For this review, take the finished solid that the model builds, in its own axes (mm). Face numbers are marked on the shaded views. A direction names the side the tool comes from. Give positions to 0.01 mm unless a question says otherwise; leave off trailing zeros. Loops run counter-clockwise (first coordinate to the right, second up) from the corner with the lowest first, then second, coordinate; pieces in that order, holes last. Notation, with made-up numbers: (17.5, 89) - (74.5, 89) arc R10 cw to (74.5, 96) - close; hole circle Ø3 at (-13, 57). An arc over 180 degrees is marked (long way). Answer as CSV lines item,"result".
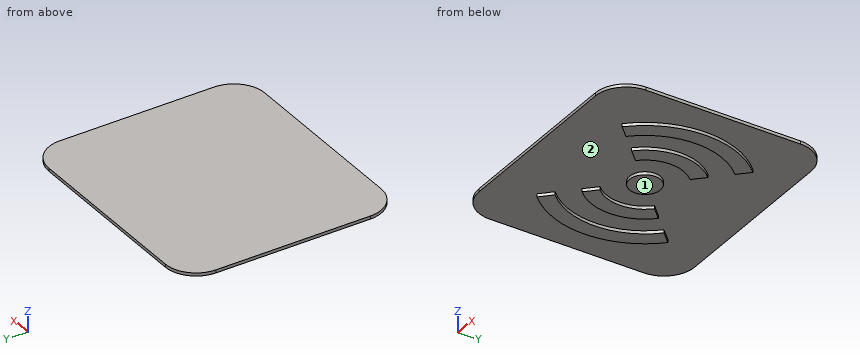
from build123d import *

# Parameters (mm, degrees)
SKETCH1_W           = 78
SKETCH1_H           = 70
BOSS_EXTRUDE1_DEPTH = 1
FILLET1_R           = 10
SKETCH2_R           = 5
BOSS_EXTRUDE3_DEPTH = 1


with BuildPart() as part:
    # Sketch1 → Boss-Extrude1 (new body)
    with BuildSketch(Plane.XY):
        with Locations((-0.075399098, 4.950190099)):
            Rectangle(SKETCH1_W, SKETCH1_H)
    extrude(amount=BOSS_EXTRUDE1_DEPTH)

    # Fillet1
    fillet1_edges = [part.edges().sort_by_distance(p)[0] for p in [
        (38.924600902, -30.049809901, 0.5),
        (-39.075399098, -30.049809901, 0.5),
        (-39.075399098, 39.950190099, 0.5),
        (38.924600902, 39.950190099, 0.5),
    ]]
    fillet(fillet1_edges, radius=FILLET1_R)

    # Sketch2 → Boss-Extrude3 (add)
    with BuildSketch(Plane(origin=(0, 0, 0), x_dir=(-1, 0, 0), z_dir=(0, 0, -1))):
        with BuildLine():
            Line((12.449767768, -7.424178572), (8.914233862, -3.888644666))
            ThreePointArc((8.914233862, -3.888644666), (12.575399098, 4.950190099), (8.914233862, 13.789024864))
            Line((8.914233862, 13.789024864), (12.449767768, 17.32455877))
            ThreePointArc((12.449767768, 17.32455877), (17.575399098, 4.950190099), (12.449767768, -7.424178572))
        make_face()
        with Locations(Location((0.075399098, 4.950190099, 0), (0, 0, 180))):
            Circle(SKETCH2_R)
        with BuildLine():
            Line((21.288602533, -16.263013337), (17.753068627, -12.727479431))
            ThreePointArc((17.753068627, -12.727479431), (25.075399098, 4.950190099), (17.753068627, 22.627859629))
            Line((17.753068627, 22.627859629), (21.288602533, 26.163393535))
            ThreePointArc((21.288602533, 26.163393535), (30.075399098, 4.950190099), (21.288602533, -16.263013337))
        make_face()
        with BuildLine():
            Line((-12.298969573, -7.424178572), (-8.763435667, -3.888644666))
            ThreePointArc((-8.763435667, -3.888644666), (-12.424600902, 4.950190099), (-8.763435667, 13.789024864))
            Line((-8.763435667, 13.789024864), (-12.298969573, 17.32455877))
            ThreePointArc((-12.298969573, 17.32455877), (-17.424600902, 4.950190099), (-12.298969573, -7.424178572))
        make_face()
        with BuildLine():
            Line((-21.137804338, -16.263013337), (-17.602270432, -12.727479431))
            ThreePointArc((-17.602270432, -12.727479431), (-24.924600902, 4.950190099), (-17.602270432, 22.627859629))
            Line((-17.602270432, 22.627859629), (-21.137804338, 26.163393535))
            ThreePointArc((-21.137804338, 26.163393535), (-29.924600902, 4.950190099), (-21.137804338, -16.263013337))
        make_face()
    extrude(amount=BOSS_EXTRUDE3_DEPTH)


solid = part.part
1) Consider section C-C on y = 21. Write out the cut boundary in (x, z).
From the geometry:
outline,"(-39.08, 0) - (-25.42, 0) - (-25.42, -1) - (-19.24, -1) - (-19.24, 0) - (19.09, 0) - (19.09, -1) - (25.27, -1) - (25.27, 0) - (38.92, 0) - (38.92, 1) - (-39.08, 1) - close"
2) Wall thickness on line 1 (X direction, y = 10.5, z = -0.6); line 2 (X direction, y = -12, z = -0.35); line 3 (Z direction, x = 20.5, y = -27): over which ranges is each line inside the solid? List them lowest first. Write a range as from..to.
From the geometry:
line 1,"x = -29.56..-24.45, -16.67..-11.28, 11.13..16.52, 24.3..29.41"
line 2,"x = -24.83..-18.45, 18.3..24.68"
line 3,"z = 0..1"
3) Consider section B-B on x = -4. Write out the cut boundary in (y, z), and give its area (3 significant figures).
From the geometry:
outline,"(-30.05, 0) - (1.85, 0) - (1.85, -1) - (8.05, -1) - (8.05, 0) - (39.95, 0) - (39.95, 1) - (-30.05, 1) - close"
area,"76.2 mm^2"
4) Consider section A-A on z = 0.55. Write out the cut boundary in (x, y), and give its area (3 significant figures).
From the geometry:
outline,"(-39.08, -20.05) arc R10 ccw to (-29.08, -30.05) - (28.92, -30.05) arc R10 ccw to (38.92, -20.05) - (38.92, 29.95) arc R10 ccw to (28.92, 39.95) - (-29.08, 39.95) arc R10 ccw to (-39.08, 29.95) - close"
area,"5,370 mm^2"
5) Insertion check: P1, Ø4, axis at x = 18.5, y = -17, coming from the -Z side. The pin has a flat end and moves straight along its axis. Give the tip position at first contact, or say it passes through.
From the geometry:
P1,"stops at z = 0"
6) Consider section D-D on x = 24. Write out the cut boundary in (y, z).
From the geometry:
outline,"(-30.05, 0) - (-12.95, 0) - (-12.95, -1) - (-1.79, -1) - (-1.79, 0) - (11.69, 0) - (11.69, -1) - (22.85, -1) - (22.85, 0) - (39.95, 0) - (39.95, 1) - (-30.05, 1) - close"
7) Machinability: for the marked faces 1 and 2, which of the approach directions +Z, -Z, +X, -X, +Y, -Y give a long, thin tool a straight path to every point of the face, cutting with its end or side? Answer none if there is none.
From the geometry:
face 1,"-Z, +X, -X, +Y, -Y"
face 2,"-Z"
